Here's the drawing with two shaded views (mm, measured from the low corner). I have some questions. Coordinates: 2 decimals unless noted, no trailing zeros. Write each loop counter-clockwise with the first axis right and the second up, starting at its lowest first coordinate (ties: lowest second). Pieces come first, ordered by that corner, then holes. Notation, with made-up numbers: (66.25, -36.75) -> (105.25, -36.75) arc R5 ccw to (105.25, -29.75) -> close; hole circle Ø3 at (-12, 53.25). An arc over 180 degrees is marked (long way). Use one line per item in the form item = value.
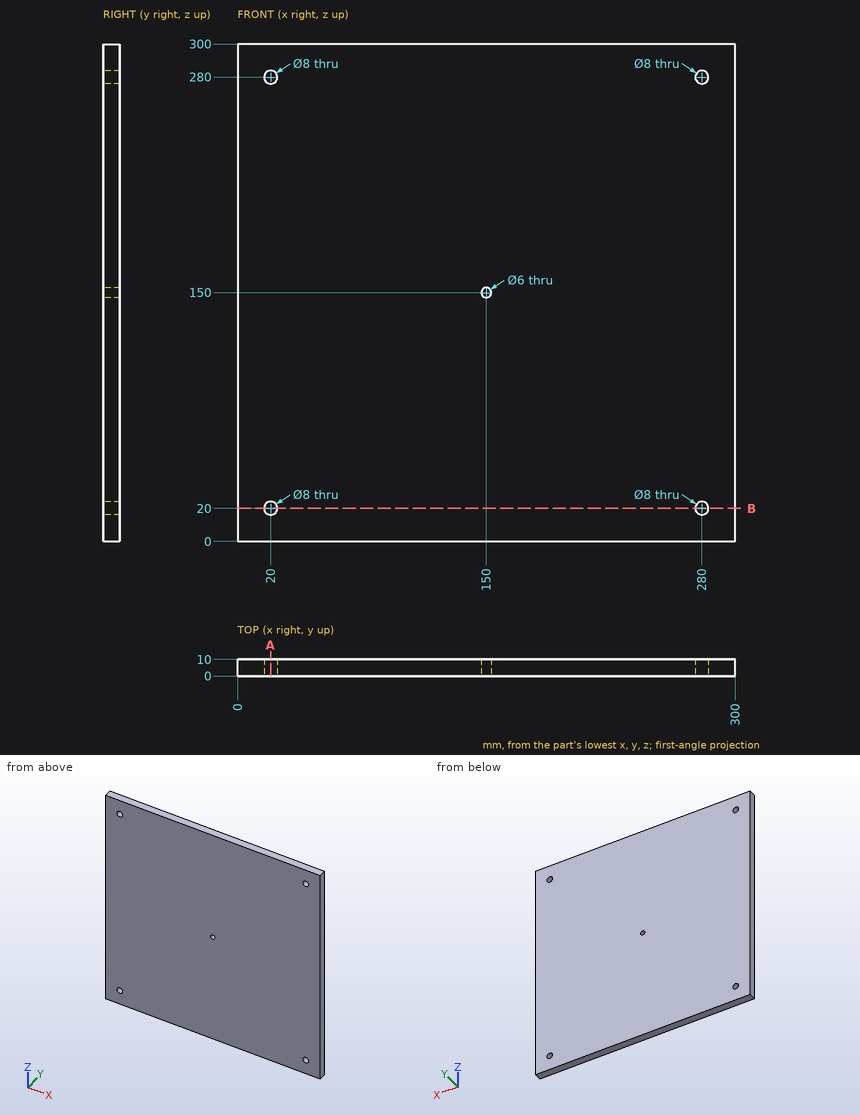
Q1. If I drill on line 1 (Z direction, x = 280, y = 5.75), over which ranges is the centre line in solid material (lowest first)? Write a range as from..to.
Return value:
line_1 = 0..16, 24..276, 284..300
Q2. Suppose I cut it at A-A (x = 20). Write out the boundary of the cut face in (y, z), then the cut area to 3 significant figures.
Return value:
outline = (0, 0) -> (10, 0) -> (10, 16) -> (0, 16) -> close; (0, 24) -> (10, 24) -> (10, 276) -> (0, 276) -> close; (0, 284) -> (10, 284) -> (10, 300) -> (0, 300) -> close
area = 2,840 mm2
Q3. Suppose I cut it at B-B (z = 20). Write out the boundary of the cut face in (x, y).
Return value:
outline = (0, 0) -> (16, 0) -> (16, 10) -> (0, 10) -> close; (24, 0) -> (276, 0) -> (276, 10) -> (24, 10) -> close; (284, 0) -> (300, 0) -> (300, 10) -> (284, 10) -> close
